Job drawing, mm, ordinate dimensions from the low corner. One solid piece. Give positions to 0.01 mm unless a question says otherwise; leave off trailing zeros. Write each loop counter-clockwise with the first axis right and the second up, starting at its lowest first coordinate (ties: lowest second). Pieces come first, ordered by that corner, then holes. Notation, with made-up numbers: (30, 76) - (84, 76) arc R23 ccw to (84, 93) - close; hole circle Ø6 at (-34.75, -4.5). An arc over 180 degrees is marked (long way). Answer in a Markdown table with one row per item. Add a question column.
1. Drop flat-ended pins along their axis: pin 1 Ø4.5 at (x, z) = (7, 36.5) entering from +Y; pin 2 Ø2 at (x, z) = (60.5, 66) entering from +Y. Give the stop position or say it passes through.
2. Probe line 1 along Z through (x, y) = (23.5, 6); line 2 along X through (y, z) = (1, 24.5); line 3 along X through (y, z) = (2, 8.5). List the from-to ranges inside material, lowest first.
3. Band-saw the part on A-A on z = 45. Write the cut outline in (x, y).
4. Band-saw the part on D-D on x = 6.5. Write the cut outline in (y, z), plus the area to 3 significant figures.
5. Band-saw the part on C-C on y = 5. Write the cut outline in (x, z).
6. Band-saw the part on B-B on x = 40.5. Write the cut outline in (y, z).
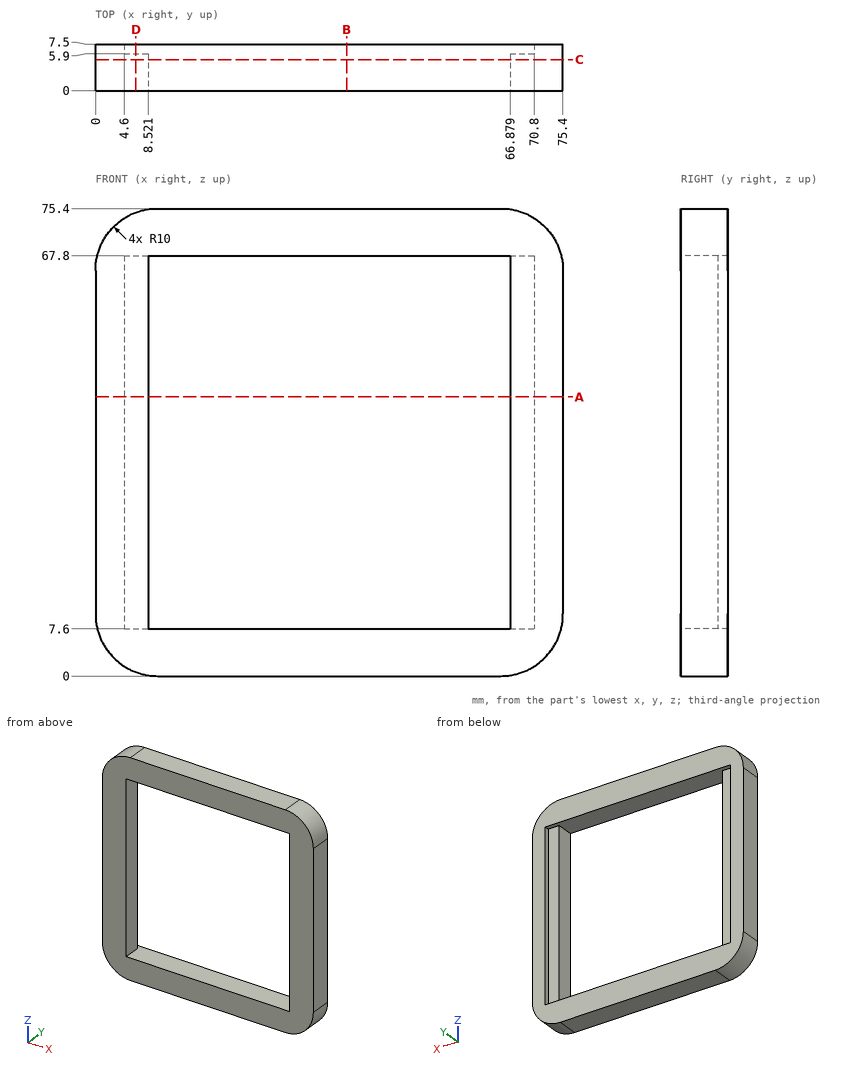
Values:
| question | item | result |
|---|---|---|
| 1 | pin 1 | stops at y = 5.9 |
| 1 | pin 2 | passes through |
| 2 | line 1 | z = 0 to 7.6, 67.8 to 75.4 |
| 2 | line 2 | x = 0 to 8.52, 66.88 to 75.4 |
| 2 | line 3 | x = 0.11 to 8.52, 66.88 to 75.29 |
| 3 | outline | (0, 0) - (8.52, 0) - (8.52, 5.9) - (4.6, 5.9) - (4.6, 7.5) - (0, 7.5) - close; (66.88, 0) - (75.4, 0) - (75.4, 7.5) - (70.8, 7.5) - (70.8, 5.9) - (66.88, 5.9) - close |
| 4 | outline | (0, 0.63) - (7.5, 0.63) - (7.5, 7.6) - (5.9, 7.6) - (5.9, 67.8) - (7.5, 67.8) - (7.5, 74.77) - (0, 74.77) - close |
| 4 | area | 460 mm² |
| 5 | outline | (0, 10) arc R10 ccw to (10, 0) - (65.4, 0) arc R10 ccw to (75.4, 10) - (75.4, 65.4) arc R10 ccw to (65.4, 75.4) - (10, 75.4) arc R10 ccw to (0, 65.4) - close; hole (8.52, 7.6) - (66.88, 7.6) - (66.88, 67.8) - (8.52, 67.8) - close |
| 6 | outline | (0, 0) - (7.5, 0) - (7.5, 7.6) - (0, 7.6) - close; (0, 67.8) - (7.5, 67.8) - (7.5, 75.4) - (0, 75.4) - close |
